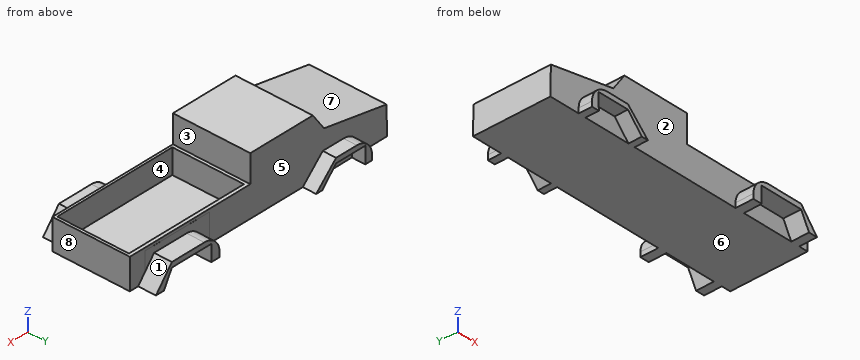
from build123d import *

# Parameters (mm, degrees)
F1_DEPTH  = 73.0149932206
F2_W      = 104.7701835632
F2_H      = 146.0299864411
F2_W_2    = 132.2311162949
F2_H_2    = 146.0643596947
F3_DEPTH  = 52.4154347368
F5_DEPTH  = 98.2172647491
F6_W      = 16.9606506824
F6_H      = 30.608355999
F7_DEPTH  = 106.583558023
F8_W      = 234.6536517143
F8_H      = 135.0331306458
F9_DEPTH  = 105.9223469347
F10_W     = 239.1506135464
F10_H     = 140.1097029448
F11_DEPTH = 11.3217700273
F12_R     = 31.0869450518


with BuildPart() as f1:
    # F0 (on Front) → F1 (new body, symmetric)
    with BuildSketch(Plane.XZ):
        Polygon((-196.8656778336, 76.734662056), (-324.1775035858, 53.8567006588), (-325.180709362, 0), (-285.0417494774, 0), (-285.0417494774, 34.4426184893), (-233.2133054733, 34.4426184893), (-232.1556210518, 0), (76.5154957771, 0), (76.5154957771, 33.5566699505), (141.2207484245, 33.5566699505), (140.163064003, 0), (199.3955373764, 0), (199.3955373764, 57.7045381069), (-46.3645458221, 57.7045381069), (-46.3645458221, 109.5087528229), (-173.955321312, 109.5087528229), align=None)
    extrude(amount=F1_DEPTH, both=True)

    # F2 (on face) → F3 (join)
    with BuildSketch(Plane(origin=(0, 0, 0), x_dir=(1, 0, 0), z_dir=(0, 0, -1))):
        with Locations((-246.2981939316, 0)):
            Rectangle(F2_W, F2_H)
        with Locations((102.5924086571, -0.0171866268)):
            Rectangle(F2_W_2, F2_H_2)
    extrude(amount=-F3_DEPTH)

    # F4 (on Front) → F5 (join, symmetric)
    with BuildSketch(Plane.XZ):
        Polygon((-194.1774785519, 40.3228625655), (-267.4925923347, 40.3228625655), (-267.4925923347, 31.2233567238), (-254.5548379421, 31.2233567238), (-194.1774785519, 31.2233567238), align=None)
        Polygon((-153.4504890442, 0), (-194.1774785519, 40.3228625655), (-194.1774785519, 31.2233567238), (-165.9055352211, 0), align=None)
        Polygon((-254.5548379421, 31.2233567238), (-267.4925923347, 31.2233567238), (-267.4925923347, 0), (-253.5964548588, 0), align=None)
    extrude(amount=F5_DEPTH, both=True)

    # F6 (on Front) → F7 (join, symmetric)
    with BuildSketch(Plane.XZ):
        Polygon((52.5457262993, 39.950683713), (52.5457262993, 30.608355999), (69.5063769817, 30.608355999), (149.9110460281, 30.608355999), (149.9110460281, 39.950683713), align=None)
        with Locations((61.0260516405, 15.3041779995)):
            Rectangle(F6_W, F6_H)
        Polygon((149.9110460281, 39.950683713), (149.9110460281, 30.608355999), (166.1303341389, 0), (182.3496222496, 0), align=None)
    extrude(amount=F7_DEPTH, both=True)

    # F8 (on Top) → F9 (cut)
    with BuildSketch(Plane.XY):
        with Locations((76.9363343716, -1.0031461716)):
            Rectangle(F8_W, F8_H)
    extrude(amount=F9_DEPTH, mode=Mode.SUBTRACT)

    # F10 (on Top) → F11 (join)
    with BuildSketch(Plane.XY):
        with Locations((76.5912085772, -0.3399476409)):
            Rectangle(F10_W, F10_H)
    extrude(amount=F11_DEPTH)

    # F12
    f12_edges = [f1.edges().sort_by_distance(p)[0] for p in [
        (52.545726, 89.816462, 39.950684),
        (-267.492592, 85.616129, 40.322863),
        (-267.492592, -85.616129, 40.322863),
        (52.545726, -89.799276, 39.950684),
    ]]
    fillet(f12_edges, radius=F12_R)


solid = f1.part
Geometry: final body of the model. Coordinates: model frame, mm. Face numbers are marked on the shaded views. A direction names the side the tool comes from. Coordinates: 2 decimals unless noted, no trailing zeros. Loops run counter-clockwise (first coordinate to the right, second up) from the corner with the lowest first, then second, coordinate; pieces in that order, holes last. Notation, with made-up numbers: (60, 65) - (73, 65) arc R24 cw to (73, 80) - close; hole circle Ø3 at (-3, -11.5). An arc over 180 degrees is marked (long way). Put each result on its own line as item: value. Start each with the question number.
Q1. Pull-direction query (X, two-part tool) for the marked faces 5, 6, 7 and 8; classes: released by +X, released by -X, zero draft, split by the parting line, or undercut.
Q2. Cut plane D-D, the plane x = 120. Return loops of the section in (y, z) (3 decimals).
Q3. Line query: line 1 (Y direction, x = 107.5, z = 47.5) (3 decimals); line 2 (Y direction, x = -73, z = 39.5) (3 decimals); line 3 (Z direction, x = -202, y = -74). Output: solid intervals per line, ascending.
Q4. Cut plane A-A, the plane x = -9.5. Return loops of the section in (y, z) (3 decimals), and give its area (3 significant figures).
Q5. Cut plane C-C, the plane z = 83. Return loops of the section in (x, y) (3 decimals), and give its area (3 significant figures).
Q6. Cut plane B-B, the plane y = -24.5. Return loops of the section in (x, z).
Q7. Set-up query: the marked faces 1, 2, 3 and 4. Return all of +Z, -Z, +X, -X, +Y, -Y with unobstructed straight access to the full face (end or side cutting, diameter ignored); none if empty.
Q8. Pin query (flat end, axial travel): pin 1 Ø12 at (x, z) = (-200, 14) entering from +Y (3 decimals); pin 2 Ø8 at (y, z) = (58, 37) entering from -X; pin 3 Ø8 at (x, y) = (8, -34.5) entering from +Z. Return the tip coordinate at first contact, or that it passes through.
Filled sheet:
1. face 5: undercut
1. face 6: zero draft
1. face 7: released by -X
1. face 8: released by +X
2. outline: (-106.584, 30.608) - (-73.015, 30.608) - (-73.015, 0) - (73.049, 0) - (73.049, 30.608) - (106.584, 30.608) - (106.584, 39.951) - (73.049, 39.951) - (73.049, 52.415) - (73.015, 52.415) - (73.015, 57.705) - (66.513, 57.705) - (66.513, 11.322) - (-68.52, 11.322) - (-68.52, 57.705) - (-73.015, 57.705) - (-73.015, 39.951) - (-106.584, 39.951) - close
3. line 1: -73.015 to -68.52, 66.513 to 73.049
3. line 2: -73.015 to 73.015
3. line 3: 31.22 to 40.32
4. outline: (-73.015, 0) - (73.015, 0) - (73.015, 57.705) - (66.513, 57.705) - (66.513, 11.322) - (-68.52, 11.322) - (-68.52, 57.705) - (-73.015, 57.705) - close
4. area: 2,160 mm²
5. outline: (-192.486, -73.015) - (-46.365, -73.015) - (-46.365, 73.015) - (-192.486, 73.015) - close
5. area: 21,300 mm²
6. outline: (-325.18, 0) - (199.4, 0) - (199.4, 57.7) - (194.26, 57.7) - (194.26, 11.32) - (-40.39, 11.32) - (-40.39, 57.7) - (-46.36, 57.7) - (-46.36, 109.51) - (-173.96, 109.51) - (-196.87, 76.73) - (-324.18, 53.86) - close
7. face 1: +Z, +X, +Y
7. face 2: +Z, -Y
7. face 3: +Z, +X, +Y, -Y
7. face 4: +Z
8. pin 1: y = 73.015
8. pin 2: x = -324.57
8. pin 3: z = 11.32
